Verification items for the finished model (mm, model axes). Face numbers are marked on the shaded views. A direction names the side the tool comes from. Give positions to 0.01 mm unless a question says otherwise; leave off trailing zeros. Order: outer loops, then holes, each group sorted by start corner. A loop starts at its lowest first (then second) coordinate and runs counter-clockwise, first axis right, second up. Notation, with made-up numbers: (-1.5, 43) - (50.5, 43) arc R14 cw to (50.5, 62) - close; hole circle Ø11 at (59, 71). An arc over 180 degrees is marked (long way). Answer as a JSON object with one key per item and string values. Group by question number.
(1) Section check C-C (y = 12.5). Record the boundary of the cut face in (x, z).
(2) Depth check by flat-ended pin: pin 1 Ø6 at (y, z) = (5.5, 11.5) entering from +X; pin 2 Ø4 at (x, y) = (15, 0) entering from +Z; pin 3 Ø6 at (x, z) = (2, 7.5) entering from +Y. Enter the tip coordinate at first touch or a pass-through.
(3) Access from +Z, -Z, +X, -X, +Y, -Y to the whole of each face (thin tool, end or side, straight path). Record for the marked faces 1, 2, 3 and 4.
(4) Section check D-D (y = 6.75). Record the boundary of the cut face in (x, z).
(5) Mould release check, pull along X, two halves, no side actions. Record for the marked faces 5, 6 and 7: +X half, -X half, draft (parallel to the pull), parting line (faces both ways), or undercut.
(6) Section check A-A (y = 4.25). Record the boundary of the cut face in (x, z).
(7) Thickness scan on line 1 (Y direction, x = 0.5, z = 10.5); line 2 (Y direction, x = 8, z = 5); line 3 (Z direction, x = 0.5, y = 4). Record the ranges inside material, lowest first.
(8) Section check B-B (x = 4). Record the boundary of the cut face in (y, z).
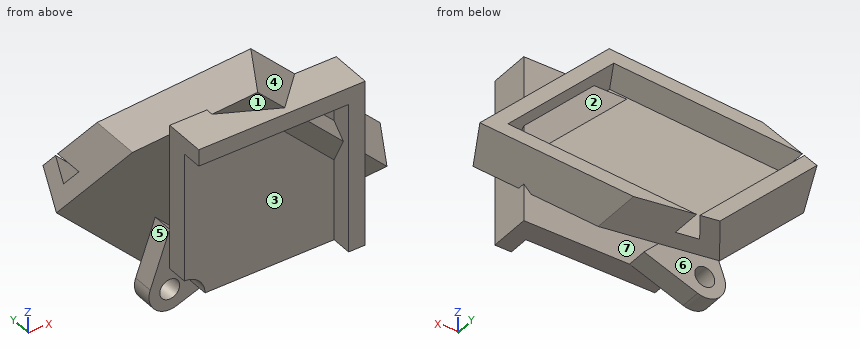
```python
from build123d import *

# Parameters (mm, degrees)
BOSS_EXTRUDE1_DEPTH      = 2.5
BOSS_EXTRUDE2_DEPTH      = 5
BOSS_EXTRUDE3_DEPTH      = 2.5
SKETCH7_W                = 22
SKETCH7_H                = 27.5
SKETCH7_W_2              = 18
SKETCH7_H_2              = 23.5
BOSS_EXTRUDE4_DEPTH      = 5
M2_CLEARANCE_HOLE1_D     = 2.4
M2_CLEARANCE_HOLE1_DEPTH = 7.5
BOSS_EXTRUDE5_DEPTH      = 2
CUT_EXTRUDE5_DEPTH       = 42.382841321


with BuildPart() as part:
    # Sketch1 → Boss-Extrude1 (new body)
    with BuildSketch(Plane(origin=(0, 0, 0), x_dir=(1, 0, 0), z_dir=(0, 1, 0))):
        with BuildLine():
            Line((0, -2.5), (0, -18.03))
            Line((0, -18.03), (18.03, -18.03))
            Line((18.03, -18.03), (18.03, 0))
            Line((18.03, 0), (2.5, 0))
            ThreePointArc((2.5, 0), (1.767766953, -1.767766953), (0, -2.5))
        make_face()
    extrude(amount=BOSS_EXTRUDE1_DEPTH)

    # Sketch2 → Boss-Extrude2 (add)
    with BuildSketch(Plane(origin=(0, 2.5, 0), x_dir=(1, 0, 0), z_dir=(0, 1, 0))):
        Polygon((0, -20.03), (0, -18.03), (18.03, -18.03), (18.03, 0), (20.03, 0), (20.03, -20.03), align=None)
    extrude(amount=-BOSS_EXTRUDE2_DEPTH)

    # Sketch3 → Boss-Extrude3 (add)
    with BuildSketch(Plane(origin=(0, 2.5, 0), x_dir=(1, 0, 0), z_dir=(0, 1, 0))):
        with BuildLine():
            Line((0.855050358, 2.349231552), (7.309511, 0))
            Line((7.309511, 0), (0, -7.309511))
            Line((0, -7.309511), (-2.349231552, -0.855050358))
            ThreePointArc((-2.349231552, -0.855050358), (-1.767766953, 1.767766953), (0.855050358, 2.349231552))
        make_face()
    extrude(amount=BOSS_EXTRUDE3_DEPTH)

    # Sketch7 → Boss-Extrude4 (add)
    with BuildSketch(Plane(origin=(6.597772224, 13.325561997, 6.597772224), x_dir=(0.7071067811865464, 0, -0.7071067811865488), z_dir=(0.40557978767264036, 0.819152044288991, 0.40557978767263897))):
        with Locations((0, -5.123791374)):
            Rectangle(SKETCH7_W, SKETCH7_H)
        with Locations((0, -5.123791374)):
            Rectangle(SKETCH7_W_2, SKETCH7_H_2, mode=Mode.SUBTRACT)
    extrude(amount=-BOSS_EXTRUDE4_DEPTH)

    # M2 Clearance Hole1
    with Locations(Plane(origin=(0, 5, 0), x_dir=(1, 0, 0), z_dir=(0, 1, 0))):
        with Locations((0, 0)):
            Hole(M2_CLEARANCE_HOLE1_D / 2, depth=M2_CLEARANCE_HOLE1_DEPTH)

    # Sketch10 → Boss-Extrude5 (add)
    with BuildSketch(Plane(origin=(4.569873286, 9.229801775, 4.569873286), x_dir=(0.9117676909005845, -0.3311545099281039, -0.24293284747866747), z_dir=(-0.40557978767264047, -0.8191520442889909, -0.40557978767263886))):
        Polygon((-13.961806263, -0.692416888), (1.91532614, 21.761239087), (19.878250921, 9.059533165), (4.001118518, -13.394122811), align=None)
    extrude(amount=-BOSS_EXTRUDE5_DEPTH)

    # Sketch13 → Cut-Extrude5 (cut, through all)
    with BuildSketch(Plane(origin=(0, 18.273352, 0), x_dir=(1, 0, 0), z_dir=(0, 1, 0))):
        Polygon((-8.346263934, -7.351506608), (-1.070246696, -14.627523847), (-5.52058621, -4.525828883), align=None)
        Polygon((7.351506608, 8.346263934), (14.627523847, 1.070246696), (4.525828883, 5.52058621), align=None)
    extrude(amount=-CUT_EXTRUDE5_DEPTH, mode=Mode.SUBTRACT)


solid = part.part
```
Solutions:
{
 "1": {"outline": "(-4.44, 6.98) - (6.98, -4.44) - (14.37, -1.18) - (15.21, -0.35) - (13.8, 1.07) - (10.1, -2.63) - (-2.63, 10.1) - (1.07, 13.8) - (-0.35, 15.21) - (-1.18, 14.37) - close"},
 "2": {"pin 1": "stops at x = 24.26", "pin 2": "stops at z = 20.4", "pin 3": "stops at y = 17.26"},
 "3": {"face 1": "-X, -Y", "face 2": "+Y", "face 3": "-Z, -X, -Y", "face 4": "+Z, +X, -Y"},
 "4": {"outline": "(-0.7, 14.85) - (14.85, -0.7) - (21.02, 5.46) - (19.6, 6.87) - (15.9, 3.18) - (3.18, 15.9) - (6.87, 19.6) - (5.46, 21.02) - close"},
 "5": {"face 5": "-X half", "face 6": "draft", "face 7": "undercut"},
 "6": {"outline": "(-2.35, 0.86) arc R2.5 ccw to (0.86, -2.35) - (7.31, 0) - (0, 7.31) - close; (1.82, 17.38) - (17.38, 1.82) - (23.54, 7.98) - (22.13, 9.4) - (18.43, 5.7) - (5.7, 18.43) - (9.4, 22.13) - (7.98, 23.54) - close; hole circle Ø2.4 at (0, 0)"},
 "7": {"line 1": "y = 0 to 2.5, 8.31 to 10.75", "line 2": "y = 0 to 2.5, 7.32 to 9.76", "line 3": "z = -2.45 to -1.09, 1.09 to 6.81"},
 "8": {"outline": "(-2.5, 18.03) - (0, 18.03) - (0, 0) - (2.5, 0) - (2.5, -1.2) - (5, -1.2) - (5, 3.31) - (2.5, 3.31) - (2.5, 18.73) - (14.18, -4.85) - (18.27, -0.8) - (17.13, 1.52) - (14.67, -0.91) - (5.93, 16.73) - (9.6, 16.73) - (8.2, 19.56) - (2.5, 19.56) - (2.5, 20.03) - (-2.5, 20.03) - close"}
}
